CAD build for the part. Positions are in the model's coordinates, mm. A direction names the side the tool comes from. Coordinates: 2 decimals unless noted, no trailing zeros. Loops run counter-clockwise (first coordinate to the right, second up) from the corner with the lowest first, then second, coordinate; pieces in that order, holes last. Notation, with made-up numbers: (-32, -15.5) -> (0, -15.5) arc R18 ccw to (0, -4.5) -> close; hole circle Ø6 at (-13.5, 58). An arc over 180 degrees is marked (long way). Return JSON: item names as keys, results as strings. Group by question number.
(1) Mould opens along X. For faces 3 (the face through (-1.27, -0.97, 19.73)), 4 (the face through (0, 2.5, 0.5)), 5 (the face through (-1, -1, 0)), 6 (the face through (-1.5, -0.5, 0.5)) say: pulls with the +X half, pulls with the -X half, needs draft (parallel to the pull), parting line crosses it, or undercut.
(2) Probe L1, parallel to Z at x = -2, y = -2.75; L2, parallel to X at y = 0.25, z = 4; L3, parallel to Y at x = -0.5, z = 20. List the from-to ranges inside material, lowest first.
(3) Tool access for faces 1 (the face through (0.583, 0.184, 38.321)), 2 (the face through (2.5, 0, 0.5)): list every direction of +Z, -Z, +X, -X, +Y, -Y with a clear straight run to the whole face (end or side of a thin tool).
(4) Saw through at A-A on z = 27.5. Write the cut outline in (x, y), then the cut area to 3 significant figures.
(5) Flat gauge pins, fed straight in: pin 1 Ø0.5 at (y, z) = (-1.5, 0.5) entering from -X; pin 2 Ø0.8 at (y, z) = (1.5, 0.5) entering from +X; pin 3 Ø4 at (y, z) = (-2.5, 24) entering from -X; pin 4 Ø1 at (x, y) = (2.5, 2.5) entering from -Z. Where does each tip first touch, or does it go through?
```python
from build123d import *

# Parameters (mm, degrees)
F3_DEPTH        = 1
F3_COPIES_COUNT = 4


# Not quite as in the source:
# - a pattern or mirror of a feature is missing from the dataset's text; its kind, count and spacing are read off the source's solid


with BuildPart() as f1:
    # F0 (on Front) → F1 (revolve)
    with BuildSketch(Plane.XZ):
        with BuildLine():
            Line((1.6, 35.6040361289), (0, 40))
            Line((0, 40), (0, 0))
            Line((0, 0), (4, 0))
            Line((4, 0), (4, 1))
            ThreePointArc((4, 1), (2.3029437252, 1.7029437252), (1.6, 3.4))
            Line((1.6, 3.4), (1.6, 35.6040361289))
        make_face()
    revolve(axis=Axis((0, 0, 20), (0, 0, 1)))

    # F2 (on Top) → F3 (cut)
    with BuildSketch(Plane.XY):
        Polygon((2.5, 0), (0, 0), (0, -2.5), (0.5, -2.5), (0.5, -0.5), (2.5, -0.5), align=None)
    f3 = extrude(amount=F3_DEPTH, mode=Mode.SUBTRACT)

    # F3_copies: F3 ×4 about axis
    f3_copies_axis = Axis((0, 0, 0), (0, 0, 1))
    for i in range(1, F3_COPIES_COUNT):
        add(f3.rotate(f3_copies_axis, i * 360 / F3_COPIES_COUNT), mode=Mode.SUBTRACT)


solid = f1.part
```
Geometry results:
{
 "1": {"face 3": "parting line crosses it", "face 4": "undercut", "face 5": "needs draft", "face 6": "undercut"},
 "2": {"L1": "0 to 1.08", "L2": "-1.58 to 1.58", "L3": "-1.52 to 1.52"},
 "3": {"face 1": "+Z", "face 2": "-Z"},
 "4": {"outline": "circle Ø3.2 at (0, 0)", "area": "8.04 mm²"},
 "5": {"pin 1": "x = -3.8", "pin 2": "x = 3.85", "pin 3": "x = -1.52", "pin 4": "z = 0"}
}
